CAD build for the part. Positions are in the model's coordinates, mm. A direction names the side the tool comes from. Round coordinates to 2 decimals unless told otherwise and drop trailing zeros. Loops run counter-clockwise (first coordinate to the right, second up) from the corner with the lowest first, then second, coordinate; pieces in that order, holes last. Notation, with made-up numbers: M 4,35.5 L 19,35.5 A7 ccw 19,47.5 Z; hole C 18,75 d4. An arc over 180 degrees is marked long. Use one line per item in the form item = value.
from build123d import *

# Parameters (mm, degrees)
F0_W     = 60
F0_H     = 25
F1_DEPTH = 2
F3_DEPTH = 25
F4_W     = 11.2
F4_H     = 4
F5_DEPTH = 2.2
F6_R     = 0.5


with BuildPart() as f1:
    # F0 (on Top) → F1 (new body)
    with BuildSketch(Plane.XY):
        with Locations((30, 12.5)):
            Rectangle(F0_W, F0_H)
    extrude(amount=F1_DEPTH)

    # F2 (on face) → F3 (join, through all)
    with BuildSketch(Plane(origin=(0, 25, 0), x_dir=(-1, 0, 0), z_dir=(0, 1, 0))):
        Polygon((-1.9529488989, 2), (-14, 8), (-46, 8), (-58.0470511011, 2), align=None)
    extrude(amount=-F3_DEPTH)

    # F4 (on face) → F5 (join)
    with BuildSketch(Plane.XY.offset(8)):
        with Locations((30, 5)):
            Rectangle(F4_W, F4_H)
        Polygon((22.7, 13.0000000004), (22.7, 11.9999999996), (22.7, 10), (37.3, 10), (37.3, 12.5), (37.3, 15), (22.7, 15), align=None)
        with Locations((30, 20)):
            Rectangle(F4_W, F4_H)
    extrude(amount=F5_DEPTH)

    # F6
    f6_edges = [f1.edges().sort_by_distance(p)[0] for p in [
        (24.4, 18, 9.1),
        (35.6, 18, 9.1),
        (22.7, 10, 9.1),
        (24.4, 3, 9.1),
        (35.6, 3, 9.1),
        (22.7, 15, 9.1),
        (35.6, 7, 9.1),
        (24.4, 7, 9.1),
        (24.4, 22, 9.1),
        (35.6, 22, 9.1),
        (37.3, 10, 9.1),
        (37.3, 15, 9.1),
    ]]
    fillet(f6_edges, radius=F6_R)


solid = f1.part
1. Probe line 1 along X through (y, z) = (12.5, 9); line 2 along Z through (x, y) = (41, 22); line 3 along Z through (x, y) = (48, 5.5). List the from-to ranges inside material, lowest first. Write a range as from..to.
Completed:
line_1 = 22.7..37.3
line_2 = 0..8
line_3 = 0..7
2. Cut at C-C on z = 5.75. Write the cut outline in (x, y), and give its area (3 significant figures).
Completed:
outline = M 9.48,0 L 50.52,0 L 50.52,25 L 9.48,25 Z
area = 1,030 mm2
3. Pull direction Y, two halves, no side cores. Call faces 1 (the face through (22.7, 13, 9)), 2 (the face through (30, 10, 9)), 3 (the face through (30, 25, 4)): +Y half, -Y half, draft (parallel to the pull), parting line (faces both ways), or undercut.
Completed:
face_1 = draft
face_2 = undercut
face_3 = +Y half
4. Cut at A-A on y = 12. Write the cut outline in (x, z), and give its area (3 significant figures).
Completed:
outline = M 0,0 L 60,0 L 60,2 L 58.05,2 L 46,8 L 37.3,8 L 37.3,10.2 L 22.7,10.2 L 22.7,8 L 14,8 L 1.95,2 L 0,2 Z
area = 416 mm2
5. Cut at D-D on x = 12.5. Write the cut outline in (y, z).
Completed:
outline = M 0,0 L 25,0 L 25,7.25 L 0,7.25 Z
6. Drop flat-ended pins along their axis: P1, Ø1.8, axis at x = 28, z = 9.5, coming from the -Y side; P2, Ø2.5, axis at y = 13.5, z = 9.5, coming from the -X side; P3, Ø1.8, axis at y = 5, z = 9.5, coming from the +X side. Give the stop position or say it passes through.
Completed:
P1 = 3
P2 = 22.7
P3 = 35.6
7. Tool access for faces 4 (the face through (29.8, 15.5, 8)), 5 (the face through (59, 13, 2)), 6 (the face through (30, 22, 9)): list every direction of +Z, -Z, +X, -X, +Y, -Y with a clear straight run to the whole face (end or side of a thin tool).
Completed:
face_4 = +Z
face_5 = +Z, +X, +Y, -Y
face_6 = +Z, +X, -X, +Y
8. Cut at B-B on y = 23.5. Write the cut outline in (x, z), and give its area (3 significant figures).
Completed:
outline = M 0,0 L 60,0 L 60,2 L 58.05,2 L 46,8 L 14,8 L 1.95,2 L 0,2 Z
area = 384 mm2
